Verification items for the finished model (mm, model axes). A direction names the side the tool comes from. Coordinates: 2 decimals unless noted, no trailing zeros. Loops run counter-clockwise (first coordinate to the right, second up) from the corner with the lowest first, then second, coordinate; pieces in that order, holes last. Notation, with made-up numbers: (48.5, 50.25) -> (65.5, 50.25) arc R15 ccw to (65.5, 76.25) -> close; hole circle Ø11 at (52.5, 84). An arc over 180 degrees is marked (long way). Write item = value, one per line.
```python
from build123d import *

# Parameters (mm, degrees)
F0_W     = 1
F0_H     = 6.8
F3_DEPTH = 1
F4_R     = 1
F5_DEPTH = 0.5


# Not quite as in the source:
# - a pattern or mirror of a feature is missing from the dataset's text; its kind, count and spacing are read off the source's solid


with BuildPart() as f1:
    # F0 (on Front) → F1 (revolve)
    with BuildSketch(Plane.XZ):
        with Locations((-0.5, 3.4)):
            Rectangle(F0_W, F0_H)
    revolve(axis=Axis((0, 0, 3.4), (0, 0, 1)))

    # F1_copies: F1 across plane


with BuildPart() as f1_1:
    add(f1.part)
    add(f1.part.mirror(Plane.XY.offset(3.65)))

    # F2 (on face) → F3 (join)
    with BuildSketch(Plane.XY.offset(6.8)):
        Polygon((1.4549226784, 0.84), (0, 1.68), (-1.4549226784, 0.84), (-1.4549226784, -0.84), (0, -1.68), (1.4549226784, -0.84), align=None)
        with BuildLine():
            ThreePointArc((1, 0), (-0.7071067812, -0.7071067812), (0, 1))
            ThreePointArc((0, 1), (0.7071067812, 0.7071067812), (1, 0))
        make_face(mode=Mode.SUBTRACT)
    extrude(amount=F3_DEPTH)

    # F4 (on face) → F5 (cut)
    with BuildSketch(Plane.XY.offset(7.8)):
        Circle(F4_R)
    extrude(amount=-F5_DEPTH, mode=Mode.SUBTRACT)


solid = f1_1.part
```
1) Tool access check on faces 5 (the face through (-0.34, -1.1, 6.8)), 6 (the face through (-0.34, -1.1, 7.8)). Record the directions out of +Z, -Z, +X, -X, +Y, -Y that give a thin tool (end or side, any length) a straight path to the whole face; none if there is none.
Ans:
face_5 = -Z
face_6 = +Z, +X, -X, +Y, -Y
2) Sectioned sample at A-A, the plane x = 0.3. Record the cut outline in (y, z).
Ans:
outline = (-1.51, 6.8) -> (-0.95, 6.8) -> (-0.95, 0) -> (0.95, 0) -> (0.95, 6.8) -> (1.51, 6.8) -> (1.51, 7.8) -> (0.95, 7.8) -> (0.95, 7.3) -> (-0.95, 7.3) -> (-0.95, 7.8) -> (-1.51, 7.8) -> close
3) Material ranges on line 1 (X direction, y = 0, z = 7.4); line 2 (Z direction, x = 0, y = 0.4); line 3 (Z direction, x = -1.3, y = 0.65), recorded low to high.
Ans:
line_1 = -1.45 to -1, 1 to 1.45
line_2 = 0 to 7.3
line_3 = 6.8 to 7.8
4) Sectioned sample at C-C, the plane y = 0.1. Record the cut outline in (x, z).
Ans:
outline = (-1.45, 6.8) -> (-0.99, 6.8) -> (-0.99, 0) -> (0.99, 0) -> (0.99, 6.8) -> (1.45, 6.8) -> (1.45, 7.8) -> (0.99, 7.8) -> (0.99, 7.3) -> (-0.99, 7.3) -> (-0.99, 7.8) -> (-1.45, 7.8) -> close
5) Sectioned sample at B-B, the plane z = 7. Record the cut outline in (x, y).
Ans:
outline = (-1.45, -0.84) -> (0, -1.68) -> (1.45, -0.84) -> (1.45, 0.84) -> (0, 1.68) -> (-1.45, 0.84) -> close
6) Depth check by flat-ended pin: pin 1 Ø2 at (y, z) = (-0.5, 3) entering from -X; pin 2 Ø1 at (x, z) = (0.5, 6) entering from +Y; pin 3 Ø2 at (y, z) = (-0.5, 3) entering from +X. Enter the tip coordinate at first touch or a pass-through.
Ans:
pin_1 = -1
pin_2 = 1
pin_3 = 1
7) Release check for a two-part mould opening along Y. For faces 1 (the face through (0, 0, 7.3)), 2 (the face through (-0.738, -1.254, 7.293)), 3 (the face through (-0.717, 1.266, 7.293)), 4 (the face through (0, 0, 0)) record: pulls with the +Y half, pulls with the -Y half, needs draft (parallel to the pull), parting line crosses it, or undercut.
Ans:
face_1 = undercut
face_2 = pulls with the -Y half
face_3 = pulls with the +Y half
face_4 = needs draft
